Geometry check sheet. Reference: the model listing, model coordinates, mm. Face numbers are marked on the shaded views. Round coordinates to 2 decimals unless told otherwise and drop trailing zeros. Write each loop counter-clockwise with the first axis right and the second up, starting at its lowest first coordinate (ties: lowest second). Pieces come first, ordered by that corner, then holes. Notation, with made-up numbers: M -39.75,41 L -29.75,41 A24 ccw -29.75,72 Z; hole C 11,-11 d9. An arc over 180 degrees is marked long. Put each result on its own line as item: value. Start each with the question number.
(1) Mould release check, pull along Y, two halves, no side actions. Record for the marked faces 1, 2 and 3: pulls with the +Y half, pulls with the -Y half, needs draft (parallel to the pull), parting line crosses it, or undercut.
(2) Section check A-A on x = -30. Record the cut outline in (y, z), then the cut area to 3 significant figures.
(3) Section check C-C on z = 9. Record the cut outline in (x, y), then the cut area to 3 significant figures.
(4) Gauge pin test, flat end, axial feed: pin 1 (1 mm diameter, centred on x = -30.5, y = -17, fed in from -Z). Record the tip position at first contact, or that the pin passes through.
(5) Material ranges on probe 1 along Y at (x, z) = (10, 3); probe 2 along X at (y, z) = (-22.5, 4); probe 3 along Y at (x, z) = (-30, 3.75), recorded low to high.
(6) Section check B-B on y = -25. Record the cut outline in (x, z).
from build123d import *

# Parameters (mm, degrees)
SKETCH_1_W                = 60
SKETCH_1_H                = 80
EXTRUDE_1_DEPTH           = 10
CHAMFER_1_SIZE            = 5
HOLE_WIZARD_9_0_9_1_D     = 9
HOLE_WIZARD_9_0_9_1_DEPTH = 34.5
HOLE_WIZARD_9_0_9_1_TIP   = 2.703872786
HOLE_WIZARD_M8_3_D        = 6.8
HOLE_WIZARD_M8_3_DEPTH    = 22.25
HOLE_WIZARD_M8_3_TIP      = 2.042926105


with BuildPart() as part:
    # 草图1 → 凸台-拉伸1 (new body)
    with BuildSketch(Plane.XY):
        with Locations((-10, 0)):
            Rectangle(SKETCH_1_W, SKETCH_1_H)
    extrude(amount=EXTRUDE_1_DEPTH)

    # 倒角1
    chamfer_1_edges = [part.edges().sort_by_distance(p)[0] for p in [
        (20, -40, 5),
        (-40, -40, 5),
        (-40, 40, 5),
        (20, 40, 5),
    ]]
    chamfer(chamfer_1_edges, length=CHAMFER_1_SIZE)

    # Ø9.0 (9) 直径孔1
    with Locations(Plane.XY.offset(10)):
        with Locations((-30, 25), (-30, -25), (-10, -25), (-10, 25)):
            Hole(HOLE_WIZARD_9_0_9_1_D / 2, depth=HOLE_WIZARD_9_0_9_1_DEPTH)
            with Locations((0, 0, -(HOLE_WIZARD_9_0_9_1_DEPTH + HOLE_WIZARD_9_0_9_1_TIP / 2))):  # 118° drill point
                Cone(0, HOLE_WIZARD_9_0_9_1_D / 2, HOLE_WIZARD_9_0_9_1_TIP, mode=Mode.SUBTRACT)

    # M8 螺纹孔3
    with Locations(Plane.XY.offset(10)):
        with Locations((10, -25), (10, 25)):
            Hole(HOLE_WIZARD_M8_3_D / 2, depth=HOLE_WIZARD_M8_3_DEPTH)
            with Locations((0, 0, -(HOLE_WIZARD_M8_3_DEPTH + HOLE_WIZARD_M8_3_TIP / 2))):  # 118° drill point
                Cone(0, HOLE_WIZARD_M8_3_D / 2, HOLE_WIZARD_M8_3_TIP, mode=Mode.SUBTRACT)


solid = part.part
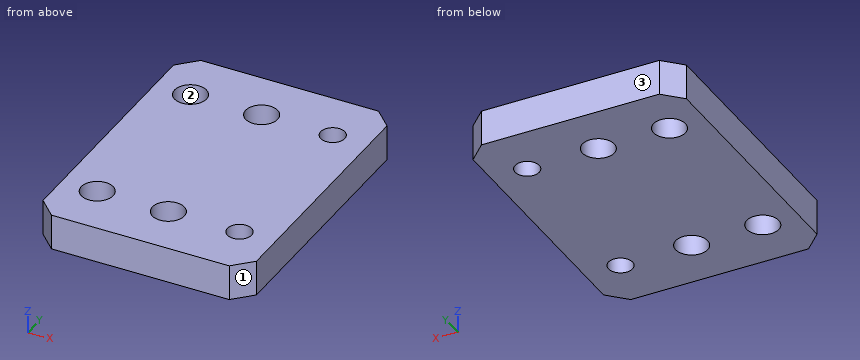
Answers follow:
1. face 1: pulls with the -Y half
1. face 2: undercut
1. face 3: pulls with the +Y half
2. outline: M -40,0 L -29.5,0 L -29.5,10 L -40,10 Z; M -20.5,0 L 20.5,0 L 20.5,10 L -20.5,10 Z; M 29.5,0 L 40,0 L 40,10 L 29.5,10 Z
2. area: 620 mm^2
3. outline: M -40,-35 L -35,-40 L 15,-40 L 20,-35 L 20,35 L 15,40 L -35,40 L -40,35 Z; hole C -30,-25 d9; hole C -30,25 d9; hole C -10,-25 d9; hole C -10,25 d9; hole C 10,-25 d6.8; hole C 10,25 d6.8
3. area: 4,420 mm^2
4. pin 1: stops at z = 0
5. probe 1: y = -40 to -28.4, -21.6 to 21.6, 28.4 to 40
5. probe 2: x = -40 to -33.74, -26.26 to -13.74, -6.26 to 7.7, 12.3 to 20
5. probe 3: y = -40 to -29.5, -20.5 to 20.5, 29.5 to 40
6. outline: M -40,0 L -34.5,0 L -34.5,10 L -40,10 Z; M -25.5,0 L -14.5,0 L -14.5,10 L -25.5,10 Z; M -5.5,0 L 6.6,0 L 6.6,10 L -5.5,10 Z; M 13.4,0 L 20,0 L 20,10 L 13.4,10 Z
